Input: part model. Units: mm. Frame: model coordinates. Face numbers are marked on the shaded views. Give positions to 0.01 mm unless a question says otherwise; leave off trailing zeros. Loops run counter-clockwise (first coordinate to the right, second up) from the corner with the lowest first, then second, coordinate; pieces in that order, holes last. Notation, with made-up numbers: M 86,82.5 L 124,82.5 A14 cw 124,91.5 Z; hole C 43.5,-30 d6. An arc over 180 degrees is marked long. One line per item, written item: value. Start each with the question number.
(1) Pull-direction query (Z, two-part tool) for the marked faces 1, 2 and 3; classes: released by +Z, released by -Z, zero draft, split by the parting line, or undercut.
(2) Section C-C on z = 2.9. Output: boundary loops of the cut face in (x, y).
(3) Section D-D on z = 1.3. Output: boundary loops of the cut face in (x, y).
(4) Pin query (flat end, axial travel): P1, Ø2, axis at x = -1.5, z = 2, coming from the -Y side; P2, Ø3, axis at x = -1, z = 5.5, coming from the -Y side; P3, Ø1.5, axis at x = 2, y = 1.5, coming from the +Z side. Return the tip coordinate at first contact, or that it passes through.
(5) Ray query, line 1 along Y through (x, z) = (-0.7, 2.45); line 2 along Y through (x, z) = (-0.85, 1.35); line 3 along X through (y, z) = (1.3, 2.85). Return the intervals inside material, ascending. Write a range as from..to.
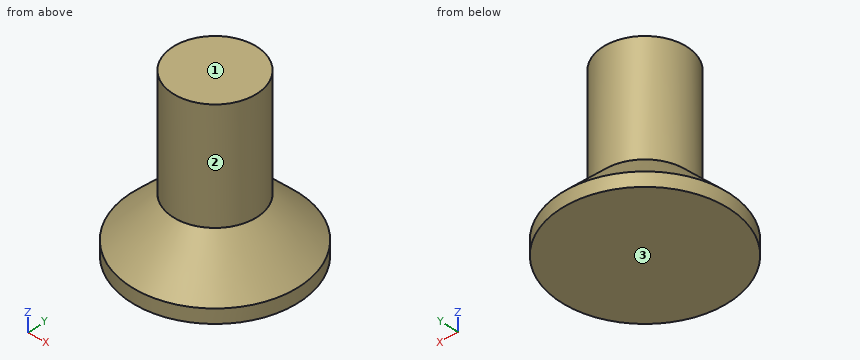
Autodesk Inventor part; units mm, degrees
ref_plane "YZ Plane" through (0, 0, 0) normal (1, 0, 0) x (0, 1, 0)
ref_plane "XZ Plane" through (0, 0, 0) normal (0, 1, 0) x (-1, 0, 0)
ref_plane "XY Plane" through (0, 0, 0) normal (0, 0, 1) x (1, 0, 0)
sketch "スケッチ1" plane through (0, 0, 0) normal (0, 0, 1) x (1, 0, 0)
  circle A0 centre (0, 0) radius 1.5
  dimension "d0" = 3
extrude "押し出し1" add sketch "スケッチ1" along normal blind 6
sketch "スケッチ2" plane through (0, 0, 0) normal (0, 0, -1) x (-1, 0, 0)
  circle A0 centre (0, 0) radius 3
  dimension "d3" = 6
extrude "押し出し2" add sketch "スケッチ2" against normal blind 2
thread "ねじ1"
chamfer "面取り1" distance 1.5 angle 45 1 edges at (3, 0, 2)
properties part number "ネジ皿m3,06" material "鋼、高強度、低合金"
Output values:
1. face 1: released by +Z
1. face 2: zero draft
1. face 3: released by -Z
2. outline: C 0,0 d3
3. outline: C 0,0 d4.4
4. P1: stops at y = -2.15
4. P2: stops at y = -1.5
4. P3: stops at z = 1.75
5. line 1: y = -1.33..1.33
5. line 2: y = -1.97..1.97
5. line 3: x = -0.75..0.75
